Can you work these out from the model? Positions are in its coordinate system, mm. A direction names the side the tool comes from. Round coordinates to 2 decimals unless told otherwise and drop trailing zeros. Loops run counter-clockwise (first coordinate to the right, second up) from the corner with the lowest first, then second, coordinate; pieces in that order, holes last.
Autodesk Inventor part; units mm, degrees
ref_plane "YZ Plane" through (0, 0, 0) normal (1, 0, 0) x (0, 1, 0)
ref_plane "XZ Plane" through (0, 0, 0) normal (0, 1, 0) x (-1, 0, 0)
ref_plane "XY Plane" through (0, 0, 0) normal (0, 0, 1) x (1, 0, 0)
sketch "Sketch5" plane through (0, 0, 0) normal (0, 0, 1) x (1, 0, 0)
  circle A0 centre (0, 0) radius 38.1
  circle A1 centre (0, 0) radius 12.7
  arc A2 (1.5875, 15.7954) -> (-1.5875, 15.7954) centre (0, 0) ccw
  line L0 (0, 0) -> (0, 15.875) construction
  line L1 (-1.5875, 15.7954) -> (-1.5875, 12.6004)
  line L2 (1.5875, 12.6004) -> (1.5875, 15.7954)
  dimension "d11" = 76.2
  dimension "d12" = 25.4
  dimension "d13" = 31.75
  dimension "d14" = 1.5875
  dimension "d15" = 1.5875
extrude "Extrusion4" add sketch "Sketch5" along normal blind 9.525
properties part number "clutch03-simplyGearDisk" material "Polycarbonate, Smoke"
(1) For faces 1 (the cylindrical face through (-0.022, 15.875, 4.696)), 2 (the flat face through (16, 1, 0)), which set-ups out of +Z, -Z, +X, -X, +Y, -Y let a thin tool reach every point of the face, with its end or its side?
Worked answers:
face 1: +Z, -Z
face 2: -Z, +X, -X, +Y, -Y
(2) If we section it at A-A, the plane y = 0: List the corners of the cut face in (x, z) for me (3 decimals), then the cut area to 3 significant figures.
Worked answers:
outline: (-38.1, 0) - (-12.7, 0) - (-12.7, 9.525) - (-38.1, 9.525) - close; (12.7, 0) - (38.1, 0) - (38.1, 9.525) - (12.7, 9.525) - close
area: 484 mm2
(3) If we section it at C-C, the plane z = 2.5: List the corners of the cut face in (x, y) for me, then the cut area to 3 significant figures.
Worked answers:
outline: circle Ø76.2 at (0, 0); hole (-1.59, 12.6) arc R12.7 ccw (long way) to (1.59, 12.6) - (1.59, 15.8) arc R15.87 ccw to (-1.59, 15.8) - close
area: 4,040 mm2
(4) If we mould it in two halves opening along Y, with no side actions, what happens to faces 3 (the cylindrical face through (-30.235, 23.183, 4.696)), 4 (the flat face through (-1.588, 14, 5)), 5 (the flat face through (16, 1, 9.525))? For each: released by +Y, released by -Y, zero draft, split by the parting line, or undercut.
Worked answers:
face 3: split by the parting line
face 4: undercut
face 5: zero draft
(5) If I drill on line 1 (Y direction, x = 0, z = 5.5); line 2 (Y direction, x = -4.5, z = 6); line 3 (X direction, y = 7.5, z = 1.25), over which ranges is the centre line in solid material (lowest first)?
Worked answers:
line 1: y = -38.1 to -12.7, 15.87 to 38.1
line 2: y = -37.83 to -11.88, 11.88 to 37.83
line 3: x = -37.35 to -10.25, 10.25 to 37.35
(6) If we section it at B-B, the plane x = 0: List the corners of the cut face in (y, z) for me (3 decimals).
Worked answers:
outline: (-38.1, 0) - (-12.7, 0) - (-12.7, 9.525) - (-38.1, 9.525) - close; (15.875, 0) - (38.1, 0) - (38.1, 9.525) - (15.875, 9.525) - close
(7) Will these pins go through, and if not, where does the flat tip stop? P1, Ø5, axis at x = -4, z = 3.5, coming from the -Y side; P2, Ø4, axis at y = -13.5, z = 3.5, coming from the -X side; P3, Ø2, axis at x = 10, z = 1.5, coming from the -Y side.
Worked answers:
P1: stops at y = -38.07
P2: stops at x = -36.32
P3: stops at y = -37.02
(8) If we section it at D-D, the plane y = 19: List the corners of the cut face in (x, z) for me (3 decimals), then the cut area to 3 significant figures.
Worked answers:
outline: (-33.024, 0) - (33.024, 0) - (33.024, 9.525) - (-33.024, 9.525) - close
area: 629 mm2
